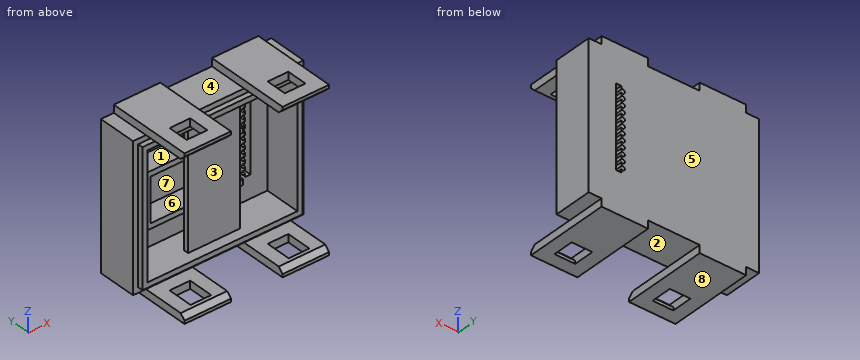
```python
from build123d import *

# Parameters (mm, degrees)
SKETCH1_W           = 66
SKETCH1_H           = 56
BASE_DEPTH          = 3
WALL1_START         = -3
SKETCH4_W           = 66
SKETCH4_H           = 56
SKETCH4_W_2         = 58
SKETCH4_H_2         = 48
WALL1_DEPTH         = 12
WALL2_START         = -15
SKETCH8_W           = 62
SKETCH8_H           = 52
SKETCH8_W_2         = 58
SKETCH8_H_2         = 48
WALL2_DEPTH         = 2
BATTERYWALL_START   = -3
BATTERYWALL_DEPTH   = 8
BATTERYHOLDER_START = -11
SKETCH10_W          = 20
SKETCH10_H          = 48
BATTERYHOLDER_DEPTH = 2
BATTERYNOTCH_START  = -3
SKETCH15_W          = 1
SKETCH15_H          = 5
BATTERYNOTCH_DEPTH  = 1.2
BATTERYNOTCH2_R     = 1
CLIPS1_START        = 28
SKETCH11_W          = 18
SKETCH11_H          = 33
SKETCH11_W_2        = 8
SKETCH11_H_2        = 8
CLIPS1_DEPTH        = 3
CLIPS2_START        = -28
SKETCH11_2_W        = 18
SKETCH11_2_H        = 33
SKETCH11_2_W_2      = 8
SKETCH11_2_H_2      = 8
CLIPS2_DEPTH        = 3
CHAMFER3_SIZE       = 1.8
WIRESLOTS_START     = -3
SKETCH12_R          = 0.8
WIRESLOTS_DEPTH     = 60.026779311
WIRESLOTS2_START    = -3
SKETCH13_W          = 2.034314575
SKETCH13_H          = 31.54
WIRESLOTS2_DEPTH    = 60.026779311


with BuildPart() as part:
    # Sketch1 → Base (new body)
    with BuildSketch(Plane(origin=(0, 0, 0), x_dir=(1, 0, 0), z_dir=(0, 1, 0))):
        Rectangle(SKETCH1_W, SKETCH1_H)
    extrude(amount=-BASE_DEPTH)

    # Sketch4 → Wall1 (add)
    with BuildSketch(Plane(origin=(0, 0, 0), x_dir=(1, 0, 0), z_dir=(0, 1, 0)).offset(WALL1_START)):
        Rectangle(SKETCH4_W, SKETCH4_H)
        Rectangle(SKETCH4_W_2, SKETCH4_H_2, mode=Mode.SUBTRACT)
    extrude(amount=-WALL1_DEPTH)

    # Sketch8 → Wall2 (add)
    with BuildSketch(Plane(origin=(0, 0, 0), x_dir=(1, 0, 0), z_dir=(0, 1, 0)).offset(WALL2_START)):
        Rectangle(SKETCH8_W, SKETCH8_H)
        Rectangle(SKETCH8_W_2, SKETCH8_H_2, mode=Mode.SUBTRACT)
    extrude(amount=-WALL2_DEPTH)

    # Sketch9 → BatteryWall (add)
    with BuildSketch(Plane(origin=(0, 0, 0), x_dir=(1, 0, 0), z_dir=(0, 1, 0)).offset(BATTERYWALL_START)):
        Polygon((-23, 8.5), (13, 8.5), (13, 10.5), (-25, 10.5), (-25, -10.5), (13, -10.5), (13, -8.5), (-23, -8.5), align=None)
    extrude(amount=-BATTERYWALL_DEPTH)

    # Sketch10 → BatteryHolder (add)
    with BuildSketch(Plane(origin=(0, 0, 0), x_dir=(1, 0, 0), z_dir=(0, 1, 0)).offset(BATTERYHOLDER_START)):
        Rectangle(SKETCH10_W, SKETCH10_H)
    extrude(amount=-BATTERYHOLDER_DEPTH)

    # Sketch15 → BatteryNotch (add)
    with BuildSketch(Plane(origin=(0, 0, 0), x_dir=(1, 0, 0), z_dir=(0, 1, 0)).offset(BATTERYNOTCH_START)):
        with Locations((13.5, 0.010715453)):
            Rectangle(SKETCH15_W, SKETCH15_H)
    extrude(amount=-BATTERYNOTCH_DEPTH)

    # BatteryNotch2
    # the kernel refuses this fillet: 1 mm, written as the material it takes off along each edge
    with BuildSketch(Plane(origin=(14, -4.2, 4.989284547), x_dir=(0, 1, 0), z_dir=(0, 0, -1)), Plane(origin=(13, -4.2, -5.010715453), x_dir=(0, 1, 0), z_dir=(0, 0, 1))) as batterynotch2_piece_1:
        with BuildLine():
            CenterArc((BATTERYNOTCH2_R, -BATTERYNOTCH2_R), BATTERYNOTCH2_R, 90, 90)
            Line((0, -BATTERYNOTCH2_R), (0, 0))
            Line((0, 0), (BATTERYNOTCH2_R, 0))
        make_face()
    extrude(amount=10, mode=Mode.SUBTRACT)
    with BuildSketch(Plane(origin=(10.5, -4.2, 2.489284547), x_dir=(0, 1, 0), z_dir=(1, 0, 0)), Plane(origin=(16.5, -4.2, -2.510715453), x_dir=(0, 1, 0), z_dir=(-1, 0, 0))) as batterynotch2_piece_2:
        with BuildLine():
            CenterArc((BATTERYNOTCH2_R, -BATTERYNOTCH2_R), BATTERYNOTCH2_R, 90, 90)
            Line((0, -BATTERYNOTCH2_R), (0, 0))
            Line((0, 0), (BATTERYNOTCH2_R, 0))
        make_face()
    extrude(amount=6, mode=Mode.SUBTRACT)

    # Sketch11 → Clips1 (add)
    # profile 1 of 2: a face of its own
    with BuildSketch(Plane.XY.offset(CLIPS1_START)):
        with Locations((-19, -16.5)):
            Rectangle(SKETCH11_W, SKETCH11_H)
        with Locations((-19, -24)):
            Rectangle(SKETCH11_W_2, SKETCH11_H_2, mode=Mode.SUBTRACT)
    # profile 2 of 2: a face of its own
    with BuildSketch(Plane.XY.offset(CLIPS1_START)):
        with Locations((19, -16.5)):
            Rectangle(SKETCH11_W, SKETCH11_H)
        with Locations((19, -24)):
            Rectangle(SKETCH11_W_2, SKETCH11_H_2, mode=Mode.SUBTRACT)
    extrude(amount=CLIPS1_DEPTH)

    # Sketch11<2> → Clips2 (add)
    # profile 1 of 2: a face of its own
    with BuildSketch(Plane.XY.offset(CLIPS2_START)):
        with Locations((-19, -16.5)):
            Rectangle(SKETCH11_2_W, SKETCH11_2_H)
        with Locations((-19, -24)):
            Rectangle(SKETCH11_2_W_2, SKETCH11_2_H_2, mode=Mode.SUBTRACT)
    # profile 2 of 2: a face of its own
    with BuildSketch(Plane.XY.offset(CLIPS2_START)):
        with Locations((19, -16.5)):
            Rectangle(SKETCH11_2_W, SKETCH11_2_H)
        with Locations((19, -24)):
            Rectangle(SKETCH11_2_W_2, SKETCH11_2_H_2, mode=Mode.SUBTRACT)
    extrude(amount=-CLIPS2_DEPTH)

    # Chamfer3
    chamfer3_edges = [part.edges().sort_by_distance(p)[0] for p in [
        (-19, -33, 28),
        (-19, -28, 28),
        (19, -33, 28),
        (19, -28, 28),
        (-19, -28, -28),
        (-19, -33, -28),
        (19, -28, -28),
        (19, -33, -28),
    ]]
    chamfer(chamfer3_edges, length=CHAMFER3_SIZE)

    # Sketch12 → WireSlots (cut, through all)
    with BuildSketch(Plane(origin=(0, 0, 0), x_dir=(1, 0, 0), z_dir=(0, 1, 0)).offset(WIRESLOTS_START)):
        with Locations(Location((19.8, -14.5, 0), (0, 0, 90))):
            Circle(SKETCH12_R)
        with Locations(Location((19.8, -11.96, 0), (0, 0, 90))):
            Circle(SKETCH12_R)
        with Locations(Location((19.8, -9.42, 0), (0, 0, 90))):
            Circle(SKETCH12_R)
        with Locations(Location((19.8, -6.88, 0), (0, 0, 90))):
            Circle(SKETCH12_R)
        with Locations(Location((19.8, -4.34, 0), (0, 0, 90))):
            Circle(SKETCH12_R)
        with Locations(Location((19.8, -1.8, 0), (0, 0, 90))):
            Circle(SKETCH12_R)
        with Locations(Location((19.8, 0.74, 0), (0, 0, 90))):
            Circle(SKETCH12_R)
        with Locations(Location((19.8, 3.28, 0), (0, 0, 90))):
            Circle(SKETCH12_R)
        with Locations(Location((19.8, 5.82, 0), (0, 0, 90))):
            Circle(SKETCH12_R)
        with Locations(Location((19.8, 8.36, 0), (0, 0, 90))):
            Circle(SKETCH12_R)
        with Locations(Location((19.8, 10.9, 0), (0, 0, 90))):
            Circle(SKETCH12_R)
        with Locations(Location((19.8, 13.44, 0), (0, 0, 90))):
            Circle(SKETCH12_R)
    extrude(amount=WIRESLOTS_DEPTH, mode=Mode.SUBTRACT)

    # Sketch13 → WireSlots2 (cut, through all)
    with BuildSketch(Plane(origin=(0, 0, 0), x_dir=(1, 0, 0), z_dir=(0, 1, 0)).offset(WIRESLOTS2_START)):
        with Locations((21.382842713, -0.53)):
            Rectangle(SKETCH13_W, SKETCH13_H)
    extrude(amount=WIRESLOTS2_DEPTH, mode=Mode.SUBTRACT)


solid = part.part
```
For this review, take the finished solid that the model builds, in its own axes (mm). Face numbers are marked on the shaded views. A direction names the side the tool comes from. Coordinates: 2 decimals unless noted, no trailing zeros. Order: outer loops, then holes, each group sorted by start corner. A loop starts at its lowest first (then second) coordinate and runs counter-clockwise, first axis right, second up. Notation, with made-up numbers: (78, -24) -> (90, -24) arc R19 cw to (90, -15) -> close; hole circle Ø9 at (16, -17.75). An arc over 180 degrees is marked (long way). Answer as CSV lines item,"result".
Q1. Draft analysis for pull direction Z (two halves, no side actions). For the marked faces 5, 6, 7 and 8, state which applies: released by +Z, released by -Z, zero draft, split by the parting line, or undercut.
Model answer:
face 5,"zero draft"
face 6,"undercut"
face 7,"undercut"
face 8,"released by -Z"
Q2. We need section B-B (x = 17.5). State the section outline as (y, z) points.
Model answer:
outline,"(-33, -31) -> (-28, -31) -> (-28, -29.8) -> (-29.8, -28) -> (-31.2, -28) -> (-33, -29.8) -> close; (-33, 29.8) -> (-31.2, 28) -> (-29.8, 28) -> (-28, 29.8) -> (-28, 31) -> (-33, 31) -> close; (-20, -31) -> (0, -31) -> (0, 31) -> (-20, 31) -> (-20, 28) -> (-15, 28) -> (-15, 26) -> (-17, 26) -> (-17, 24) -> (-3, 24) -> (-3, -24) -> (-17, -24) -> (-17, -26) -> (-15, -26) -> (-15, -28) -> (-20, -28) -> close"
Q3. Clearance check with flat-ended pins moving along their axes: pin 1 Ø16.5 at (x, y) = (0.5, -8) entering from +Z; pin 2 Ø0.9 at (y, z) = (-23, 29) entering from +X; pin 3 Ø2.5 at (y, z) = (-13.5, 29.5) entering from -X. State where each tip first meets the part, or that it passes through.
Model answer:
pin 1,"stops at z = 28"
pin 2,"stops at x = 28"
pin 3,"stops at x = -28"
Q4. Wall thickness on line 1 along X through (y, z) = (-12.5, -19); line 2 along Y through (x, z) = (-7.5, -15.5); line 3 along Z through (x, y) = (20.5, -18): over which ranges is each line inside the solid? List them lowest first. Write a range as [from, to].
Model answer:
line 1,"x = [-33, -29], [-10, 10], [29, 33]"
line 2,"y = [-13, -11], [-3, 0]"
line 3,"z = [-31, -28], [28, 31]"
Q5. For the marked faces 1, 2, 3 and 4, list the 3-axis set-ups (+Z, -Z, +X, -X, +Y, -Y) from which the entire face can be reached by the end or side of a thin tool; tool diameter is ignored.
Model answer:
face 1,"none"
face 2,"-Z, +Y, -Y"
face 3,"-Y"
face 4,"+Z, +Y, -Y"
Q6. We need section D-D (x = 26.5). State the section outline as (y, z) points, plus the area to 3 significant figures.
Model answer:
outline,"(-33, -31) -> (0, -31) -> (0, 31) -> (-33, 31) -> (-33, 29.8) -> (-31.2, 28) -> (-15, 28) -> (-15, 26) -> (-17, 26) -> (-17, 24) -> (-3, 24) -> (-3, -24) -> (-17, -24) -> (-17, -26) -> (-15, -26) -> (-15, -28) -> (-31.2, -28) -> (-33, -29.8) -> close"
area,"467 mm2"
Q7. We need section A-A (y = -8). Count the separate pieces of the cut face and the enclosed holes in it, plus the area to 3 significant figures.
Model answer:
separate pieces,"2"
enclosed holes,"1"
area,"1,310 mm2"
Q8. We need section C-C (x = -7.5). State the section outline as (y, z) points, plus the area to 3 significant figures.
Model answer:
outline,"(-17, -26) -> (-15, -26) -> (-15, -28) -> (0, -28) -> (0, 28) -> (-15, 28) -> (-15, 26) -> (-17, 26) -> (-17, 24) -> (-13, 24) -> (-13, -24) -> (-17, -24) -> close; hole (-11, -24) -> (-3, -24) -> (-3, -10.5) -> (-11, -10.5) -> close; hole (-11, -8.5) -> (-3, -8.5) -> (-3, 8.5) -> (-11, 8.5) -> close; hole (-11, 10.5) -> (-3, 10.5) -> (-3, 24) -> (-11, 24) -> close"
area,"400 mm2"
